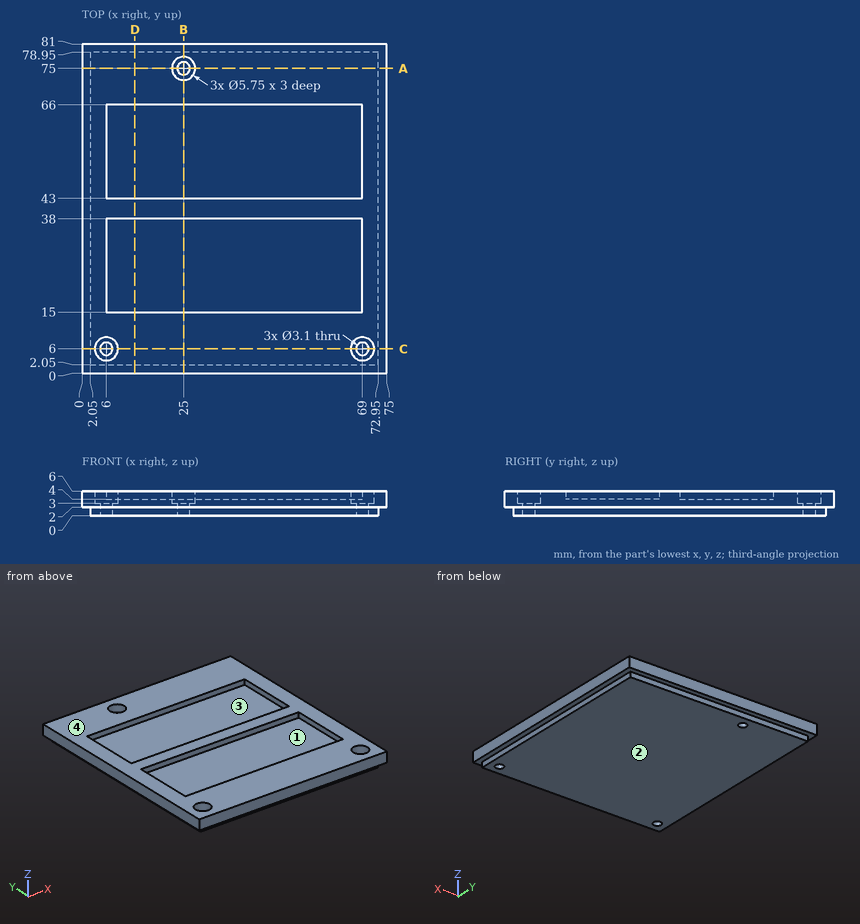
Can you work these out from the drawing? Everything is in mm from the part's minimum corner. A direction names the side the tool comes from. Give positions to 0.01 mm unless a question says otherwise; leave off trailing zeros. Order: outer loops, then holes, each group sorted by start corner. A loop starts at its lowest first (then second) coordinate and runs counter-clockwise, first axis right, second up.
Item 1: If we section it at B-B, the plane x = 25: Write out the boundary of the cut face in (y, z) (3 decimals), plus the area to 3 significant figures.
Item 2: If we section it at A-A, the plane y = 75: Write out the boundary of the cut face in (x, z) (3 decimals), plus the area to 3 significant figures.
Item 3: If we mould it in two halves opening along X, with no side actions, what happens to the marked faces 3 and 4? For each: pulls with the +X half, pulls with the -X half, needs draft (parallel to the pull), parting line crosses it, or undercut.
Item 4: If we section it at D-D, the plane x = 13: Write out the boundary of the cut face in (y, z), plus the area to 3 significant figures.
Item 5: If we section it at C-C, the plane y = 6: Write out the boundary of the cut face in (x, z) (3 decimals), plus the area to 3 significant figures.
Item 6: For the marked faces 1 and 2, which set-ups out of +Z, -Z, +X, -X, +Y, -Y let a thin tool reach every point of the face, with its end or its side?
Item 7: I'm going to push flat-ended pins straight in: pin 1 (1 mm diameter, centred on x = 30, y = 24, fed in from +Z); pin 2 (2.5 mm diameter, centred on x = 6, y = 6, fed in from -Z); pin 3 (1 mm diameter, centred on x = 55, z = 0.5, fed in from -Y). Where does each tip first touch, or does it pass through?
Item 8: I need wall thicknesses on line 1 (X direction, y = 6, z = 0.9); line 2 (Y direction, x = 34.5, z = 5.6); line 3 (X direction, y = 6, z = 4.8) (3 decimals). Which ranges of each line are inside material? Lowest first, please.
Values:
1. outline: (0, 2) - (2.05, 2) - (2.05, 0) - (73.45, 0) - (73.45, 3) - (72.125, 3) - (72.125, 6) - (66, 6) - (66, 4) - (43, 4) - (43, 6) - (38, 6) - (38, 4) - (15, 4) - (15, 6) - (0, 6) - close; (76.55, 0) - (78.95, 0) - (78.95, 2) - (81, 2) - (81, 6) - (77.875, 6) - (77.875, 3) - (76.55, 3) - close
1. area: 359 mm2
2. outline: (0, 2) - (2.05, 2) - (2.05, 0) - (23.45, 0) - (23.45, 3) - (22.125, 3) - (22.125, 6) - (0, 6) - close; (26.55, 0) - (72.95, 0) - (72.95, 2) - (75, 2) - (75, 6) - (27.875, 6) - (27.875, 3) - (26.55, 3) - close
2. area: 415 mm2
3. face 3: undercut
3. face 4: needs draft
4. outline: (0, 2) - (2.05, 2) - (2.05, 0) - (78.95, 0) - (78.95, 2) - (81, 2) - (81, 6) - (66, 6) - (66, 4) - (43, 4) - (43, 6) - (38, 6) - (38, 4) - (15, 4) - (15, 6) - (0, 6) - close
4. area: 386 mm2
5. outline: (0, 2) - (2.05, 2) - (2.05, 0) - (4.45, 0) - (4.45, 3) - (3.125, 3) - (3.125, 6) - (0, 6) - close; (7.55, 0) - (67.45, 0) - (67.45, 3) - (66.125, 3) - (66.125, 6) - (8.875, 6) - (8.875, 3) - (7.55, 3) - close; (70.55, 0) - (72.95, 0) - (72.95, 2) - (75, 2) - (75, 6) - (71.875, 6) - (71.875, 3) - (70.55, 3) - close
5. area: 389 mm2
6. face 1: +Z
6. face 2: -Z, +X, -X, +Y, -Y
7. pin 1: stops at z = 4
7. pin 2: passes through
7. pin 3: stops at y = 2.05
8. line 1: x = 2.05 to 4.45, 7.55 to 67.45, 70.55 to 72.95
8. line 2: y = 0 to 15, 38 to 43, 66 to 81
8. line 3: x = 0 to 3.125, 8.875 to 66.125, 71.875 to 75
